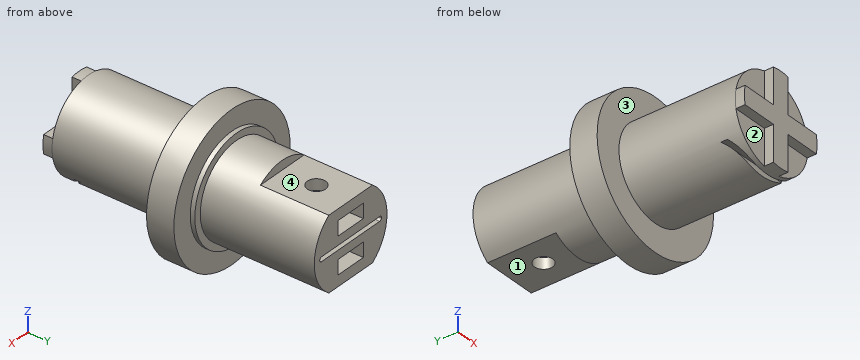
```python
from build123d import *

# Parameters (mm, degrees)
SKETCH_2_W               = 17
SKETCH_2_H               = 1
CUT_EXTRUDE_1_DEPTH      = 26
FILLET_1_R               = 0.5
CUT_EXTRUDE_START        = -15
CUT_EXTRUDE_2_DEPTH      = 15
CUT_EXTRUDE_3_DEPTH      = 15
SKETCH_5_R               = 2
CUT_EXTRUDE_4_DEPTH      = 17
EXTRUDE_START            = 2
EXTRUDE_1_DEPTH          = 2
CUT_EXTRUDE_5_DEPTH      = 8
CUT_EXTRUDE_5_DEPTH_BACK = 8


with BuildPart() as part:
    # 草图1 → 旋转1 (revolve)
    with BuildSketch(Plane.XY, mode=Mode.PRIVATE) as revolve_1_sk:
        Polygon((5, 2.5), (5, 60), (-5, 60), (-5, 35), (-6.5, 35), (-6.5, 34), (-11, 34), (-11, 28), (-5, 28), (-5, 2.5), align=None)
    revolve(revolve_1_sk.sketch.rotate(Axis((5, 2.5, 0), (0, 1, 0)), 270), axis=Axis((5, 2.5, 0), (0, 1, 0)))

    # 草图2 → 切除-拉伸1 (cut)
    with BuildSketch(Plane(origin=(0, 60, 0), x_dir=(1, 0, 0), z_dir=(0, 1, 0))):
        with Locations((5, 0)):
            Rectangle(SKETCH_2_W, SKETCH_2_H)
    extrude(amount=-CUT_EXTRUDE_1_DEPTH, mode=Mode.SUBTRACT)

    # 圆角1
    fillet_1_edges = [part.edges().sort_by_distance(p)[0] for p in [
        (-3.5, 47, 0.5),
        (-3.5, 47, -0.5),
        (13.5, 47, 0.5),
        (13.5, 47, -0.5),
    ]]
    fillet(fillet_1_edges, radius=FILLET_1_R - 0.0001)  # a hair under: the kernel refuses the full size

    # 草图3 → 切除-拉伸2 (cut)
    with BuildSketch(Plane(origin=(0, 60, 0), x_dir=(1, 0, 0), z_dir=(0, 1, 0)).offset(CUT_EXTRUDE_START)):
        with BuildLine():
            Line((5, -8), (11, -8))
            ThreePointArc((11, -8), (5, -10), (-1, -8))
            Line((-1, -8), (5, -8))
        make_face()
        with BuildLine():
            Line((5, 8), (11, 8))
            ThreePointArc((11, 8), (5, 10), (-1, 8))
            Line((-1, 8), (5, 8))
        make_face()
    extrude(amount=CUT_EXTRUDE_2_DEPTH, mode=Mode.SUBTRACT)

    # 草图4 → 切除-拉伸3 (cut)
    with BuildSketch(Plane(origin=(0, 60, 0), x_dir=(1, 0, 0), z_dir=(0, 1, 0))):
        Polygon((1.5, -2.4), (1.5, -4), (1.5, -5.6), (8.5, -5.6), (8.5, -2.4), align=None)
        Polygon((1.5, 4), (1.5, 2.4), (8.5, 2.4), (8.5, 5.6), (1.5, 5.6), align=None)
    extrude(amount=-CUT_EXTRUDE_3_DEPTH, mode=Mode.SUBTRACT)

    # 草图5 → 切除-拉伸4 (cut)
    with BuildSketch(Plane(origin=(0, 0, -8), x_dir=(-1, 0, 0), z_dir=(0, 0, -1))):
        with Locations((-5, 52.5)):
            Circle(SKETCH_5_R)
    extrude(amount=-CUT_EXTRUDE_4_DEPTH, mode=Mode.SUBTRACT)

    # 草图6 → 凸台-拉伸1 (add)
    with BuildSketch(Plane.XZ.offset(-2.5).offset(EXTRUDE_START)):
        with BuildLine():
            Line((7, 2), (14.797958971, 2))
            ThreePointArc((14.797958971, 2), (15, 0), (14.797958971, -2))
            Line((14.797958971, -2), (7, -2))
            Line((7, -2), (7, -9.797958971))
            ThreePointArc((7, -9.797958971), (5, -10), (3, -9.797958971))
            Line((3, -9.797958971), (3, -2))
            Line((3, -2), (-4.797958971, -2))
            ThreePointArc((-4.797958971, -2), (-5, 0), (-4.797958971, 2))
            Line((-4.797958971, 2), (3, 2))
            Line((3, 2), (3, 9.797958971))
            ThreePointArc((3, 9.797958971), (5, 10), (7, 9.797958971))
            Line((7, 9.797958971), (7, 2))
        make_face()
    extrude(amount=-EXTRUDE_1_DEPTH)

    # 草图7 → 切除-拉伸5 (cut, two sides: drawn at the far end of the back side and taken through both)
    with BuildSketch(Plane(origin=(5, 0, 0), x_dir=(0, 0, -1), z_dir=(1, 0, 0)).offset(-CUT_EXTRUDE_5_DEPTH_BACK)):
        with BuildLine():
            Line((10, 4.510210526), (10, 3.510210526))
            add(Edge.make_bspline(
                [(-0.5, 34), (-0.5, 3.510210526), (10, 3.510210526)],
                knots=[1.570796327, 1.570796327, 1.570796327, 3.141592654, 3.141592654, 3.141592654], degree=2, weights=[1, 0.707106781, 1]))
            Line((-0.5, 34), (0.5, 34))
            add(Edge.make_bspline(
                [(0.5, 34), (0.5, 4.510210526), (10, 4.510210526)],
                knots=[1.570796327, 1.570796327, 1.570796327, 3.141592654, 3.141592654, 3.141592654], degree=2, weights=[1, 0.707106781, 1]))
        make_face()
    extrude(amount=CUT_EXTRUDE_5_DEPTH + CUT_EXTRUDE_5_DEPTH_BACK, mode=Mode.SUBTRACT)


solid = part.part
```
Read the model definition and answer for the solid it produces. Units are mm, in the model's axes. Face numbers are marked on the shaded views. A direction names the side the tool comes from. Give positions to 0.01 mm unless a question says otherwise; leave off trailing zeros. Loops run counter-clockwise (first coordinate to the right, second up) from the corner with the lowest first, then second, coordinate; pieces in that order, holes last.
Item 1: Each of these flat-tipped pins is pushed along its axis until it touches: pin 1 Ø4 at (x, z) = (0, 6.5) entering from -Y; pin 2 Ø2 at (x, y) = (-1, 52) entering from +Z; pin 3 Ø2 at (x, z) = (14.5, 7.5) entering from +Y. Where does it stop, or does it pass through?
Item 2: Find the intervals of material crossed by line 1 along Y through (x, z) = (5, 1); line 2 along Y through (x, z) = (5, -6); line 3 along Y through (x, z) = (-5.5, -5), in increasing order.
Item 3: The part is cut by section C-C (z = -12.5). Write down the section's boundary in (x, y), and give its area (3 significant figures).
Item 4: For the marked faces 1, 2, 3 and 4, determine the directions among +Z, -Z, +X, -X, +Y, -Y from which every point of the face is accessible in a straight line to the end or side of a thin tool.
Item 5: The part is cut by section A-A (z = 7). Write down the section's boundary in (x, y).
Item 6: The part is cut by section B-B (z = 13.5). Write down the section's boundary in (x, y).
Taken from the geometry:
1. pin 1: stops at y = 2.5
1. pin 2: stops at z = 8
1. pin 3: stops at y = 35
2. line 1: y = 0.5 to 50.5, 54.5 to 60
2. line 2: y = 0.5 to 5.81, 7.25 to 50.5, 54.5 to 60
2. line 3: y = 28 to 34
3. outline: (-4.99, 28) - (14.99, 28) - (14.99, 34) - (-4.99, 34) - close
3. area: 120 mm2
4. face 1: -Z, +X, -X, +Y
4. face 2: -Z, -X, -Y
4. face 3: -Y
4. face 4: +Z, +X, -X, +Y
5. outline: (-9.39, 28) - (-2.14, 28) - (-2.14, 2.5) - (3, 2.5) - (3, 0.5) - (7, 0.5) - (7, 2.5) - (12.14, 2.5) - (12.14, 28) - (19.39, 28) - (19.39, 34) - (14.12, 34) - (14.12, 35) - (12.14, 35) - (12.14, 60) - (-2.14, 60) - (-2.14, 35) - (-4.12, 35) - (-4.12, 34) - (-9.39, 34) - close; hole circle Ø4 at (5, 52.5)
6. outline: (-3.59, 28) - (13.59, 28) - (13.59, 34) - (-3.59, 34) - close
